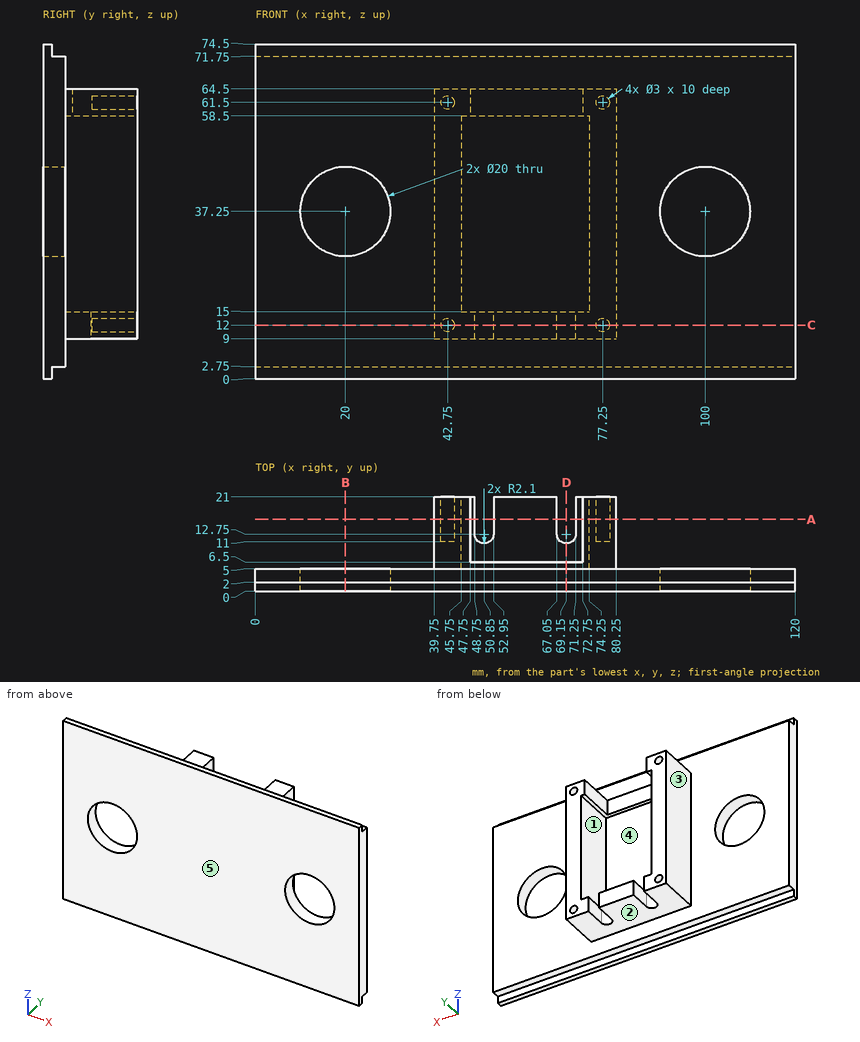
Here's the drawing with two shaded views (mm, measured from the low corner). I have some questions. A direction names the side the tool comes from. Coordinates: 2 decimals unless noted, no trailing zeros. Loops run counter-clockwise (first coordinate to the right, second up) from the corner with the lowest first, then second, coordinate; pieces in that order, holes last. Notation, with made-up numbers: (13.25, 46.25) -> (38.25, 46.25) arc R7 ccw to (38.25, 58.25) -> close; hole circle Ø2 at (-27, 3). An arc over 180 degrees is marked (long way). Put each result on its own line as item: value. Start each with the question number.
Q1. For the marked faces 4 and 5, which set-ups out of +Z, -Z, +X, -X, +Y, -Y let a thin tool reach every point of the face, with its end or its side?
Q2. I want a section at A-A (y = 16). Write out the boundary of the cut face in (x, z).
Q3. Thinking about a two-plate mould opening in Z: for the marked faces 1, 2 and 3, which applies, pulls with the +Z half, pulls with the -Z half, needs draft (parallel to the pull), parting line crosses it, or undercut?
Q4. I want a section at C-C (z = 12). Write out the boundary of the cut face in (x, y).
Q5. I'm going to push flat-ended pins straight in: P1, Ø8, axis at y = 14, z = 47.5, coming from the -X side; P2, Ø1.5, axis at x = 43, z = 12.5, coming from the +Y side; P3, Ø5, axis at x = 65.5, y = 8, coming from the -Z side. Where does each tip first touch, or does it pass through?
Q6. I want a section at B-B (x = 20). Write out the boundary of the cut face in (y, z).
Q7. I want a section at D-D (x = 69.15). Write out the boundary of the cut face in (y, z), plus the area to 3 significant figures.
Q8. If I drill on line 1 (Z direction, x = 77.25, y = 16.75); line 2 (X direction, y = 1.1, z = 37.25); line 3 (X direction, y = 9, z = 17.5), over which ranges is the centre line in solid material (lowest first)? Write a range as [from, to].
Taken from the geometry:
1. face 4: +Y
1. face 5: +Z, -Z, +X, -X, -Y
2. outline: (39.75, 9) -> (48.75, 9) -> (48.75, 15) -> (45.75, 15) -> (45.75, 58.5) -> (47.75, 58.5) -> (47.75, 64.5) -> (39.75, 64.5) -> close; (52.95, 9) -> (67.05, 9) -> (67.05, 15) -> (52.95, 15) -> close; (71.25, 9) -> (80.25, 9) -> (80.25, 64.5) -> (72.75, 64.5) -> (72.75, 58.5) -> (74.25, 58.5) -> (74.25, 15) -> (71.25, 15) -> close; hole circle Ø3 at (42.75, 12); hole circle Ø3 at (42.75, 61.5); hole circle Ø3 at (77.25, 12); hole circle Ø3 at (77.25, 61.5)
3. face 1: undercut
3. face 2: pulls with the -Z half
3. face 3: needs draft
4. outline: (0, 0) -> (120, 0) -> (120, 5) -> (80.25, 5) -> (80.25, 21) -> (78.75, 21) -> (78.75, 11) -> (75.75, 11) -> (75.75, 21) -> (71.25, 21) -> (71.25, 12.75) arc R2.1 cw to (67.05, 12.75) -> (67.05, 21) -> (52.95, 21) -> (52.95, 12.75) arc R2.1 cw to (48.75, 12.75) -> (48.75, 21) -> (44.25, 21) -> (44.25, 11) -> (41.25, 11) -> (41.25, 21) -> (39.75, 21) -> (39.75, 5) -> (0, 5) -> close
5. P1: stops at x = 39.75
5. P2: stops at y = 11
5. P3: stops at z = 9
6. outline: (0, 0) -> (2, 0) -> (2, 2.75) -> (5, 2.75) -> (5, 27.25) -> (0, 27.25) -> close; (0, 47.25) -> (5, 47.25) -> (5, 71.75) -> (2, 71.75) -> (2, 74.5) -> (0, 74.5) -> close
7. outline: (0, 0) -> (2, 0) -> (2, 2.75) -> (5, 2.75) -> (5, 9) -> (10.65, 9) -> (10.65, 15) -> (5, 15) -> (5, 58.5) -> (6.5, 58.5) -> (6.5, 64.5) -> (5, 64.5) -> (5, 71.75) -> (2, 71.75) -> (2, 74.5) -> (0, 74.5) -> close
7. area: 399 mm2
8. line 1: z = [9, 10.5], [13.5, 60], [63, 64.5]
8. line 2: x = [0, 10], [30, 90], [110, 120]
8. line 3: x = [39.75, 45.75], [74.25, 80.25]
